from build123d import *

# Parameters (mm, degrees)
CROQUIS1_W              = 73
CROQUIS1_H              = 69
CROQUIS1_R              = 3.1
CROQUIS1_R_2            = 1.5
SALIENTE_EXTRUIR1_DEPTH = 6
CROQUIS2_R              = 2.75
CORTAR_EXTRUIR1_DEPTH   = 3


with BuildPart() as part:
    # Croquis1 → Saliente-Extruir1 (new body)
    with BuildSketch(Plane.XY):
        with Locations((36.5, 34.5)):
            Rectangle(CROQUIS1_W, CROQUIS1_H)
        with Locations((6.5, 6.5)):
            Circle(CROQUIS1_R, mode=Mode.SUBTRACT)
        with Locations((66.5, 6.5)):
            Circle(CROQUIS1_R, mode=Mode.SUBTRACT)
        with Locations((66.5, 62.5)):
            Circle(CROQUIS1_R, mode=Mode.SUBTRACT)
        with Locations((6.5, 62.5)):
            Circle(CROQUIS1_R, mode=Mode.SUBTRACT)
        with Locations((18.5, 50.5)):
            Circle(CROQUIS1_R_2, mode=Mode.SUBTRACT)
        with Locations((54.5, 50.5)):
            Circle(CROQUIS1_R_2, mode=Mode.SUBTRACT)
        with Locations((54.5, 18.5)):
            Circle(CROQUIS1_R_2, mode=Mode.SUBTRACT)
        with Locations((18.5, 18.5)):
            Circle(CROQUIS1_R_2, mode=Mode.SUBTRACT)
    extrude(amount=SALIENTE_EXTRUIR1_DEPTH)

    # Croquis2 → Cortar-Extruir1 (cut)
    with BuildSketch(Plane(origin=(0, 0, 0), x_dir=(-1, 0, 0), z_dir=(0, 0, -1))):
        with Locations((-54.5, 50.5)):
            Circle(CROQUIS2_R)
        with Locations((-18.5, 50.5)):
            Circle(CROQUIS2_R)
        with Locations((-18.5, 18.5)):
            Circle(CROQUIS2_R)
        with Locations((-54.5, 18.5)):
            Circle(CROQUIS2_R)
    extrude(amount=-CORTAR_EXTRUIR1_DEPTH, mode=Mode.SUBTRACT)


solid = part.part
The listing builds one solid part. Answer for the finished solid, in the listing's coordinates (mm). A direction names the side the tool comes from. Round coordinates to 2 decimals unless told otherwise and drop trailing zeros. Order: outer loops, then holes, each group sorted by start corner. A loop starts at its lowest first (then second) coordinate and runs counter-clockwise, first axis right, second up. Notation, with made-up numbers: M 8.25,-1 L 60.25,-1 A34 ccw 60.25,35 Z; hole C 61.25,56.25 d3. An arc over 180 degrees is marked long. Answer in a Markdown table with one row per item. Add a question column.
1) Determine the mould class of faces 1 (the face through (36, 69, 3)), 2 (the face through (57.247, 18.621, 1.479)), 3 (the face through (36, 0, 3)), 4 (the face through (36, 35, 6)) for opening direction Y: pulls with the +Y half, pulls with the -Y half, needs draft (parallel to the pull), parting line crosses it, or undercut.
2) The part is cut by section A-A on x = 6.5. Determine the outline of the cut face in (y, z).
3) The part is cut by section C-C on y = 18.5. Determine the outline of the cut face in (x, z).
4) Consider line 1 along Y through (x, z) = (54.5, 2.3); line 2 along Y through (x, z) = (18.5, 4.3); line 3 along X through (y, z) = (18.5, 3.6). Determine where each line is inside the solid, lowest interval first. Write a range as from..to.
5) Which of the six approach directions +Z, -Z, +X, -X, +Y, -Y give full straight-line access (tool end or side, diameter ignored) to faces 5 (the face through (69.457, 7.431, 2.958)), 6 (the face through (56.527, 52.359, 1.479))?
6) A flat-ended cylindrical pin translates along its axis: pin 1 Ø4 at (x, y) = (54.5, 18.5) entering from -Z. Find the tip coordinate at first contact, or state that the pin passes through.
7) The part is cut by section D-D on x = 18.5. Determine the outline of the cut face in (y, z).
8) The part is cut by section B-B on z = 4.35. Count the separate pieces of the cut face and the enclosed holes in it, plus the area to 3 significant figures.
Findings below:
| question | item | result |
|---|---|---|
| 1 | face 1 | pulls with the +Y half |
| 1 | face 2 | undercut |
| 1 | face 3 | pulls with the -Y half |
| 1 | face 4 | needs draft |
| 2 | outline | M 0,0 L 3.4,0 L 3.4,6 L 0,6 Z; M 9.6,0 L 59.4,0 L 59.4,6 L 9.6,6 Z; M 65.6,0 L 69,0 L 69,6 L 65.6,6 Z |
| 3 | outline | M 0,0 L 15.75,0 L 15.75,3 L 17,3 L 17,6 L 0,6 Z; M 20,3 L 21.25,3 L 21.25,0 L 51.75,0 L 51.75,3 L 53,3 L 53,6 L 20,6 Z; M 56,3 L 57.25,3 L 57.25,0 L 73,0 L 73,6 L 56,6 Z |
| 4 | line 1 | y = 0..15.75, 21.25..47.75, 53.25..69 |
| 4 | line 2 | y = 0..17, 20..49, 52..69 |
| 4 | line 3 | x = 0..17, 20..53, 56..73 |
| 5 | face 5 | +Z, -Z |
| 5 | face 6 | -Z |
| 6 | pin 1 | stops at z = 3 |
| 7 | outline | M 0,0 L 15.75,0 L 15.75,3 L 17,3 L 17,6 L 0,6 Z; M 20,3 L 21.25,3 L 21.25,0 L 47.75,0 L 47.75,3 L 49,3 L 49,6 L 20,6 Z; M 52,3 L 53.25,3 L 53.25,0 L 69,0 L 69,6 L 52,6 Z |
| 8 | separate pieces | 1 |
| 8 | enclosed holes | 8 |
| 8 | area | 4,890 mm² |
